The listing builds one solid part. Answer for the finished solid, in the listing's coordinates (mm). Round coordinates to 2 decimals unless told otherwise and drop trailing zeros. Write each loop counter-clockwise with the first axis right and the second up, starting at its lowest first coordinate (ties: lowest second). Pieces come first, ordered by that corner, then holes. Notation, with made-up numbers: (88, 57.5) - (115, 57.5) arc R13 cw to (115, 75.5) - close; hole circle Ø10 at (12.25, -25). An arc over 180 degrees is marked (long way). Answer as CSV lines item,"result". Start each with the question number.
Item 1: Straight lines are drawn through the part: line 1 along Z through (x, y) = (76, 2.1); line 2 along X through (y, z) = (5.4, 48); line 3 along X through (y, z) = (4, 12). For each, find the intervals that lie inside material, in ascending order. Write a range as [from, to].
Item 2: A cutting plane is placed at A-A on z = -77.5. Determine the outline of the cut face in (x, y), and give its area (3 significant figures).
Item 3: Flat-ended cylindrical pins translate along their axes: pin 1 (3 mm diameter, centred on y = 3, z = -14.5, fed in from +X); pin 2 (1.8 mm diameter, centred on y = 4.5, z = -11.5, fed in from -X); pin 3 (1.8 mm diameter, centred on x = 142.5, y = 2.5, fed in from +Z); pin 4 (1 mm diameter, centred on x = 28.5, z = 31, fed in from +Y). Find the tip coordinate at first contact, or state that the pin passes through.
Item 4: A cutting plane is placed at C-C on y = 3.55. State how many separate pieces and enclosed holes the cut face has, and give its area (3 significant figures).
Item 5: A cutting plane is placed at B-B on x = 11. Determine the outline of the cut face in (y, z), and give its area (3 significant figures).
Item 6: A cutting plane is placed at D-D on z = 24. Determine the outline of the cut face in (x, y).
```python
from build123d import *

# Parameters (mm, degrees)
ESBO_O1_W                  = 150
ESBO_O1_H                  = 150
RESSALTO_EXTRUS_O1_DEPTH   = 6
ESBO_O3_W                  = 30
ESBO_O3_H                  = 6
RESSALTO_EXTRUS_O3_DEPTH   = 6
ESBO_O6_W                  = 30
ESBO_O6_H                  = 6
RESSALTO_EXTRUS_O6_DEPTH   = 6
ESBO_O7_W                  = 30
ESBO_O7_H                  = 6
RESSALTO_EXTRUS_O8_DEPTH   = 6
ESBO_O9_W                  = 90
ESBO_O9_H                  = 6
RESSALTO_EXTRUS_O9_DEPTH   = 6
ESBO_O10_W                 = 90
ESBO_O10_H                 = 6
RESSALTO_EXTRUS_O10_DEPTH  = 90
ESBO_O11_W                 = 10
ESBO_O11_H                 = 6
CORTE_EXTRUS_O1_DEPTH      = 221.698889893
CORTE_EXTRUS_O2_DEPTH      = 221.698889893
CORTE_EXTRUS_O2_DEPTH_BACK = 221.698889893
ESBO_O12_W                 = 6
ESBO_O12_H                 = 10


with BuildPart() as part:
    # Esboço1 → Ressalto-extrusão1 (new body)
    with BuildSketch(Plane(origin=(0, 0, 0), x_dir=(1, 0, 0), z_dir=(0, 1, 0))):
        with Locations((75, 75)):
            Rectangle(ESBO_O1_W, ESBO_O1_H)
    extrude(amount=RESSALTO_EXTRUS_O1_DEPTH)

    # Esboço3 → Ressalto-extrusão3 (add)
    with BuildSketch(Plane(origin=(0, 0, -150), x_dir=(-1, 0, 0), z_dir=(0, 0, -1))):
        with Locations((-105, 3)):
            Rectangle(ESBO_O3_W, ESBO_O3_H)
        with Locations((-45, 3)):
            Rectangle(ESBO_O3_W, ESBO_O3_H)
    extrude(amount=RESSALTO_EXTRUS_O3_DEPTH)

    # Esboço6 → Ressalto-extrusão6 (add)
    with BuildSketch(Plane(origin=(150, 0, 0), x_dir=(0, 0, -1), z_dir=(1, 0, 0))):
        with Locations((45, 3)):
            Rectangle(ESBO_O6_W, ESBO_O6_H)
        with Locations((105, 3)):
            Rectangle(ESBO_O6_W, ESBO_O6_H)
    extrude(amount=RESSALTO_EXTRUS_O6_DEPTH)

    # Esboço7 → Ressalto-extrusão8 (add)
    with BuildSketch(Plane.ZY):
        with Locations((-105, 3)):
            Rectangle(ESBO_O7_W, ESBO_O7_H)
        with Locations((-45, 3)):
            Rectangle(ESBO_O7_W, ESBO_O7_H)
    extrude(amount=RESSALTO_EXTRUS_O8_DEPTH)

    # Esboço9 → Ressalto-extrusão9 (add)
    with BuildSketch(Plane.XY):
        with Locations((75, 3)):
            Rectangle(ESBO_O9_W, ESBO_O9_H)
    extrude(amount=RESSALTO_EXTRUS_O9_DEPTH)

    # Esboço10 → Ressalto-extrusão10 (add)
    with BuildSketch(Plane.XY.offset(6)):
        with Locations((75, 3)):
            Rectangle(ESBO_O10_W, ESBO_O10_H)
    extrude(amount=RESSALTO_EXTRUS_O10_DEPTH)

    # Esboço11 → Corte-extrusão1 (cut, through all)
    with BuildSketch(Plane(origin=(0, 6, 0), x_dir=(1, 0, 0), z_dir=(0, 1, 0))):
        with Locations((75, -48)):
            Rectangle(ESBO_O11_W, ESBO_O11_H)
    extrude(amount=-CORTE_EXTRUS_O1_DEPTH, mode=Mode.SUBTRACT)

    # Esboço12 → Corte-extrusão2 (cut, two sides: drawn at the far end of the back side and taken through both)
    with BuildSketch(Plane(origin=(0, 6, 0), x_dir=(1, 0, 0), z_dir=(0, 1, 0)).offset(-CORTE_EXTRUS_O2_DEPTH_BACK)):
        with Locations((75, 75)):
            Rectangle(ESBO_O12_W, ESBO_O12_H)
    extrude(amount=CORTE_EXTRUS_O2_DEPTH + CORTE_EXTRUS_O2_DEPTH_BACK, mode=Mode.SUBTRACT)


solid = part.part
```
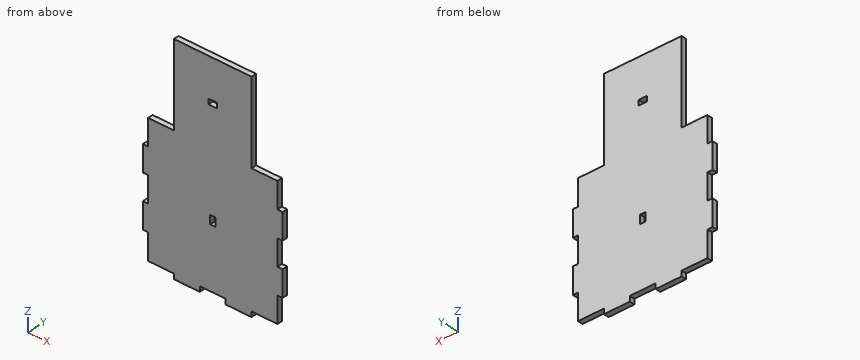
Geometry says:
1,line 1,"z = [-150, -80], [-70, 45], [51, 96]"
1,line 2,"x = [30, 70], [80, 120]"
1,line 3,"x = [30, 120]"
2,outline,"(0, 0) - (72, 0) - (72, 6) - (0, 6) - close; (78, 0) - (150, 0) - (150, 6) - (78, 6) - close"
2,area,"864 mm^2"
3,pin 1,"stops at x = 150"
3,pin 2,"stops at x = 0"
3,pin 3,"stops at z = 0"
3,pin 4,"passes through"
4,separate pieces,"1"
4,enclosed holes,"2"
4,area,"32,100 mm^2"
5,outline,"(0, -150) - (6, -150) - (6, 0) - (0, 0) - close"
5,area,"900 mm^2"
6,outline,"(30, 0) - (120, 0) - (120, 6) - (30, 6) - close"
